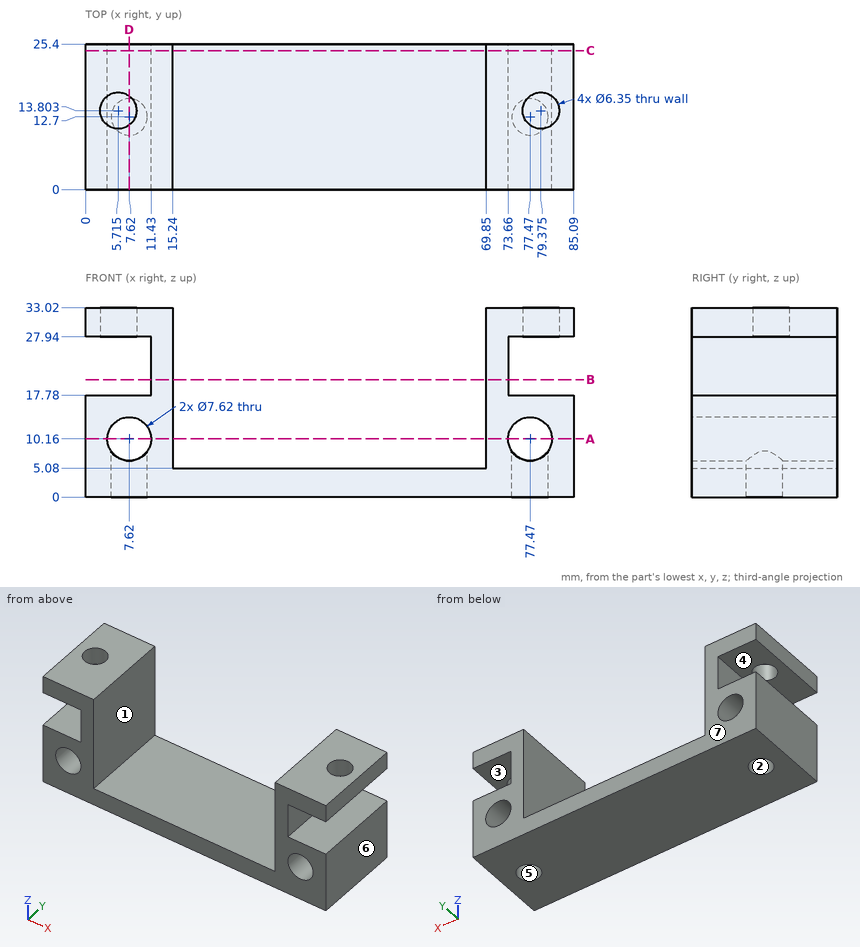
Input: dimensioned drawing with shaded views. Units: mm. Origin: part minimum x, y, z. A direction names the side the tool comes from. Coordinates: 2 decimals unless noted, no trailing zeros. Order: outer loops, then holes, each group sorted by start corner. A loop starts at its lowest first (then second) coordinate and runs counter-clockwise, first axis right, second up. Notation, with made-up numbers: (-32.75, -29.5) -> (16.25, -29.5) arc R20 ccw to (16.25, -14.5) -> close; hole circle Ø3 at (16.5, -1). An arc over 180 degrees is marked (long way). Answer in a Markdown table with one row per item.
Item 1: Access query for the marked faces 1, 2, 3 and 4. Directions: +Z, -Z, +X, -X, +Y, -Y. A direction counts if a zero-diameter tool reaches every point of the face in a straight line with its end or side. Return the directions, or none.
Return value:
| item | result |
|---|---|
| face 1 | +Z, +Y, -Y |
| face 2 | -Z |
| face 3 | +X, +Y, -Y |
| face 4 | -X, +Y, -Y |
Item 2: Ray query, L1, parallel to Z at x = 77.47, y = 20; L2, parallel to X at y = 14, z = 5; L3, parallel to Z at x = 10.5, y = 7.5 (1 decimal). Return the intervals inside material, ascending.
Return value:
| item | result |
|---|---|
| L1 | z = 0 to 6.35, 13.97 to 17.78, 27.94 to 33.02 |
| L2 | x = 0 to 4.72, 10.52 to 74.57, 80.37 to 85.09 |
| L3 | z = 0 to 7.7, 12.7 to 17.8, 27.9 to 33 |
Item 3: Section B-B on z = 20.5. Output: boundary loops of the cut face in (x, y), plus the area to 3 significant figures.
Return value:
| item | result |
|---|---|
| outline | (11.43, 0) -> (15.24, 0) -> (15.24, 25.4) -> (11.43, 25.4) -> close; (69.85, 0) -> (73.66, 0) -> (73.66, 25.4) -> (69.85, 25.4) -> close |
| area | 194 mm² |
Item 4: Section C-C on y = 24.25. Output: boundary loops of the cut face in (x, z).
Return value:
| item | result |
|---|---|
| outline | (0, 0) -> (85.09, 0) -> (85.09, 17.78) -> (73.66, 17.78) -> (73.66, 27.94) -> (85.09, 27.94) -> (85.09, 33.02) -> (69.85, 33.02) -> (69.85, 5.08) -> (15.24, 5.08) -> (15.24, 33.02) -> (0, 33.02) -> (0, 27.94) -> (11.43, 27.94) -> (11.43, 17.78) -> (0, 17.78) -> close; hole circle Ø7.62 at (7.62, 10.16); hole circle Ø7.62 at (77.47, 10.16) |
Item 5: Draft query along Y for the marked faces 5, 6 and 7. Return one class per face: released by +Y, released by -Y, zero draft, split by the parting line, or undercut.
Return value:
| item | result |
|---|---|
| face 5 | undercut |
| face 6 | zero draft |
| face 7 | released by +Y |
Item 6: Section D-D on x = 7.62. State how many separate pieces and enclosed holes the cut face has, plus the area to 3 significant figures.
Return value:
| item | result |
|---|---|
| separate pieces | 5 |
| enclosed holes | 0 |
| area | 321 mm² |
Item 7: Contact query for a flat-ended pin moving along its axis: P1, Ø3.5, axis at x = 5, y = 13.5, coming from the +Z side. Output: stop coordinate, or through.
Return value:
| item | result |
|---|---|
| P1 | stops at z = 17.78 |
Item 8: Section A-A on z = 10.16. Output: boundary loops of the cut face in (x, y).
Return value:
| item | result |
|---|---|
| outline | (0, 0) -> (3.81, 0) -> (3.81, 25.4) -> (0, 25.4) -> close; (11.43, 0) -> (15.24, 0) -> (15.24, 25.4) -> (11.43, 25.4) -> close; (69.85, 0) -> (73.66, 0) -> (73.66, 25.4) -> (69.85, 25.4) -> close; (81.28, 0) -> (85.09, 0) -> (85.09, 25.4) -> (81.28, 25.4) -> close |
